Read the model definition and answer for the solid it produces. Units are mm, in the model's axes. A direction names the side the tool comes from. Give positions to 0.01 mm unless a question says otherwise; leave off trailing zeros. Write each loop counter-clockwise with the first axis right and the second up, starting at its lowest first coordinate (ties: lowest second). Pieces come first, ordered by that corner, then holes.
```python
from build123d import *

# Parameters (mm, degrees)
BOSS_EXTRUDE1_DEPTH = 1.5
SKETCH3_W           = 9.15
SKETCH3_H           = 19
CUT_EXTRUDE1_DEPTH  = 1.5
SKETCH2_W           = 33.8
SKETCH2_H           = 1.5
BOSS_EXTRUDE2_DEPTH = 21.85
SKETCH4_R           = 1.5
CUT_EXTRUDE2_DEPTH  = 1.5
BOSS_EXTRUDE3_DEPTH = 1.5
CUT_EXTRUDE4_REACH  = 72.71
SKETCH6_R           = 1.5
SKETCH6_3_R         = 4
CUT_EXTRUDE5_DEPTH  = 1.5
SKETCH8_W           = 24
SKETCH8_H           = 23
BOSS_EXTRUDE5_DEPTH = 1.5
SKETCH9_W           = 8.5
SKETCH9_H           = 8.5
BOSS_EXTRUDE6_DEPTH = 2.7


with BuildPart() as part:
    # Sketch1 → Boss-Extrude1 (new body)
    with BuildSketch(Plane.XY):
        Polygon((-16.9, 0), (16.9, 0), (16.9, 4), (19.2, 4), (19.2, 30), (16.9, 30), (16.9, 34), (13, 34), (13, 36.4), (-13, 36.4), (-13, 34), (-16.9, 34), (-16.9, 30), (-19.2, 30), (-19.2, 4), (-16.9, 4), align=None)
    extrude(amount=BOSS_EXTRUDE1_DEPTH)

    # Sketch3 → Cut-Extrude1 (cut)
    with BuildSketch(Plane.XY.offset(1.5)):
        with Locations((0.125, 21.5)):
            Rectangle(SKETCH3_W, SKETCH3_H)
    extrude(amount=-CUT_EXTRUDE1_DEPTH, mode=Mode.SUBTRACT)

    # Sketch2 → Boss-Extrude2 (add)
    with BuildSketch(Plane(origin=(0, 0, 0), x_dir=(-1, 0, 0), z_dir=(0, 0, -1))):
        with Locations((0, 35.65)):
            Rectangle(SKETCH2_W, SKETCH2_H)
    extrude(amount=BOSS_EXTRUDE2_DEPTH)

    # Sketch4 → Cut-Extrude2 (cut)
    with BuildSketch(Plane(origin=(0, 36.4, 0), x_dir=(1, 0, 0), z_dir=(0, 1, 0))):
        with Locations(Location((-11, 11.7, 0), (0, 0, 270))):
            Circle(SKETCH4_R)
        with Locations(Location((0, 11.7, 0), (0, 0, 270))):
            Circle(SKETCH4_R)
        with Locations(Location((11, 11.7, 0), (0, 0, 270))):
            Circle(SKETCH4_R)
        with BuildLine():
            Line((-11.9, 8.25), (11.9, 8.25))
            ThreePointArc((11.9, 8.25), (13.4, 6.75), (11.9, 5.25))
            Line((11.9, 5.25), (-11.9, 5.25))
            ThreePointArc((-11.9, 5.25), (-13.4, 6.75), (-11.9, 8.25))
        make_face()
        with BuildLine():
            Line((-11.9, 18.15), (11.9, 18.15))
            ThreePointArc((11.9, 18.15), (13.4, 16.65), (11.9, 15.15))
            Line((11.9, 15.15), (-11.9, 15.15))
            ThreePointArc((-11.9, 15.15), (-13.4, 16.65), (-11.9, 18.15))
        make_face()
    extrude(amount=-CUT_EXTRUDE2_DEPTH, mode=Mode.SUBTRACT)

    # Sketch5 → Boss-Extrude3 (add)
    with BuildSketch(Plane(origin=(19.2, 0, 0), x_dir=(0, 0, -1), z_dir=(1, 0, 0))):
        Polygon((0, 30), (0.75, 30), (0.75, 34), (13.17, 46.3), (37.17, 46.3), (37.17, 20.3), (19.75, 0), (0.75, 0), (0.75, 4), (0, 4), (-1.5, 4), (-1.5, 30), align=None)
    boss_extrude3 = extrude(amount=-BOSS_EXTRUDE3_DEPTH)

    # Mirror1: Boss-Extrude3 across plane
    add(boss_extrude3.mirror(Plane(origin=(0, 0, 0), x_dir=(0, 0, 1), z_dir=(1, 0, 0))))

    # Cut-Extrude4: up to this face of the body (flat: up to its plane)
    cut_extrude4_end = Plane(part.part.faces().sort_by_distance((-19.2, 23.875362989, -17.45186466))[0])
    # Sketch6 → Cut-Extrude4 (cut, up to the picked face)
    with BuildSketch(Plane(origin=(19.2, 0, 0), x_dir=(0, 0, -1), z_dir=(1, 0, 0)), mode=Mode.PRIVATE) as cut_extrude4_sk1:
        with Locations((16.67, 42.3)):
            Circle(SKETCH6_R)
    cut_extrude4_tool1 = split(extrude(cut_extrude4_sk1.sketch, amount=-CUT_EXTRUDE4_REACH, mode=Mode.PRIVATE), bisect_by=cut_extrude4_end, keep=Keep.BOTH, mode=Mode.PRIVATE)
    # Sketch6 → Cut-Extrude4 (cut, up to the picked face)
    with BuildSketch(Plane(origin=(19.2, 0, 0), x_dir=(0, 0, -1), z_dir=(1, 0, 0)), mode=Mode.PRIVATE) as cut_extrude4_sk2:
        with Locations((24.67, 42.3)):
            Circle(SKETCH6_R)
    cut_extrude4_tool2 = split(extrude(cut_extrude4_sk2.sketch, amount=-CUT_EXTRUDE4_REACH, mode=Mode.PRIVATE), bisect_by=cut_extrude4_end, keep=Keep.BOTH, mode=Mode.PRIVATE)
    # Sketch6 → Cut-Extrude4 (cut, up to the picked face)
    with BuildSketch(Plane(origin=(19.2, 0, 0), x_dir=(0, 0, -1), z_dir=(1, 0, 0)), mode=Mode.PRIVATE) as cut_extrude4_sk3:
        with Locations((32.67, 42.3)):
            Circle(SKETCH6_R)
    cut_extrude4_tool3 = split(extrude(cut_extrude4_sk3.sketch, amount=-CUT_EXTRUDE4_REACH, mode=Mode.PRIVATE), bisect_by=cut_extrude4_end, keep=Keep.BOTH, mode=Mode.PRIVATE)
    add(cut_extrude4_tool1.solids().sort_by(Axis((19.2, 42.3, -16.67), (-1, 0, 0)))[0], mode=Mode.SUBTRACT)
    add(cut_extrude4_tool2.solids().sort_by(Axis((19.2, 42.3, -24.67), (-1, 0, 0)))[0], mode=Mode.SUBTRACT)
    add(cut_extrude4_tool3.solids().sort_by(Axis((19.2, 42.3, -32.67), (-1, 0, 0)))[0], mode=Mode.SUBTRACT)

    # Sketch6<3> → Cut-Extrude5 (cut)
    with BuildSketch(Plane(origin=(19.2, 0, 0), x_dir=(0, 0, -1), z_dir=(1, 0, 0))):
        with Locations((23.037930183, 16.5)):
            Circle(SKETCH6_3_R)
    extrude(amount=-CUT_EXTRUDE5_DEPTH, mode=Mode.SUBTRACT)

    # Sketch8 → Boss-Extrude5 (add)
    with BuildSketch(Plane(origin=(0, 0, 0), x_dir=(-1, 0, 0), z_dir=(0, 0, -1))):
        with Locations((-0.7, 20)):
            Rectangle(SKETCH8_W, SKETCH8_H)
    extrude(amount=BOSS_EXTRUDE5_DEPTH)

    # Sketch9 → Boss-Extrude6 (add)
    with BuildSketch(Plane.XY):
        with Locations((0.097336639, 16.75)):
            Rectangle(SKETCH9_W, SKETCH9_H)
    extrude(amount=BOSS_EXTRUDE6_DEPTH)


solid = part.part
```
Item 1: Determine the mould class of faces 1 (the flat face through (-16.9, 32, 1)), 2 (the flat face through (0, 36, -21.85)), 3 (the cylindrical face through (-13.4, 35.7, -16.6)) for opening direction Z: pulls with the +Z half, pulls with the -Z half, needs draft (parallel to the pull), parting line crosses it, or undercut.
Result set:
face 1: needs draft
face 2: pulls with the -Z half
face 3: undercut
Item 2: Section B-B (z = -24) is taken. Write down the section's boundary in (x, y).
Result set:
outline: (-19.2, 4.95) - (-17.7, 4.95) - (-17.7, 40.96) - (-19.2, 40.96) - close; (-19.2, 43.64) - (-17.7, 43.64) - (-17.7, 46.3) - (-19.2, 46.3) - close; (17.7, 4.95) - (19.2, 4.95) - (19.2, 12.62) - (17.7, 12.62) - close; (17.7, 20.38) - (19.2, 20.38) - (19.2, 40.96) - (17.7, 40.96) - close; (17.7, 43.64) - (19.2, 43.64) - (19.2, 46.3) - (17.7, 46.3) - close
Item 3: Find the intervals of material crossed by line 1 along X through (y, z) = (35.25, -11.7); line 2 along X through (y, z) = (15, -29); line 3 along Y through (x, z) = (18.35, -16.67), in increasing order.
Result set:
line 1: x = -19.2 to -17.7, -16.9 to -12.5, -9.5 to -1.5, 1.5 to 9.5, 12.5 to 16.9, 17.7 to 19.2
line 2: x = -19.2 to -17.7, 17.7 to 19.2
line 3: y = 0 to 40.8, 43.8 to 46.3
Item 4: Section A-A (x = 7.5) is taken. Write down the section's boundary in (y, z).
Result set:
outline: (0, 0) - (8.5, 0) - (8.5, -1.5) - (31.5, -1.5) - (31.5, 0) - (34.9, 0) - (34.9, -5.25) - (36.4, -5.25) - (36.4, 1.5) - (0, 1.5) - close; (34.9, -21.85) - (36.4, -21.85) - (36.4, -18.15) - (34.9, -18.15) - close; (34.9, -15.15) - (36.4, -15.15) - (36.4, -8.25) - (34.9, -8.25) - close
Item 5: Section C-C (y = 42.3) is taken. Give the number of separate pieces and of enclosed holes in the cut face, and give its area (3 significant figures).
Result set:
separate pieces: 8
enclosed holes: 0
area: 57.1 mm2
Item 6: Section D-D (z = -32.67) is taken. Write down the section's boundary in (x, y).
Result set:
outline: (-19.2, 15.06) - (-17.7, 15.06) - (-17.7, 40.8) - (-19.2, 40.8) - close; (-19.2, 43.8) - (-17.7, 43.8) - (-17.7, 46.3) - (-19.2, 46.3) - close; (17.7, 15.06) - (19.2, 15.06) - (19.2, 40.8) - (17.7, 40.8) - close; (17.7, 43.8) - (19.2, 43.8) - (19.2, 46.3) - (17.7, 46.3) - close
Item 7: Which of the six approach directions +Z, -Z, +X, -X, +Y, -Y give full straight-line access (tool end or side, diameter ignored) to faces 4 (the flat face through (18, 4, 0)), 5 (the cylindrical face through (13.4, 35.7, -16.7)), 6 (the flat face through (0, 21, 1))?
Result set:
face 4: +Z, +X, -Y
face 5: +Y, -Y
face 6: +Z
Item 8: Each of these flat-tipped pins is pushed along its axis until it touches: pin 1 Ø1.6 at (y, z) = (32.5, 1) entering from +X; pin 2 Ø1.2 at (x, z) = (-4, -0.5) entering from +Y; pin 3 Ø5 at (y, z) = (42.3, -24.67) entering from +X; pin 4 Ø1.1 at (x, z) = (17.5, 0) entering from +Y. Where does it stop, or does it pass through?
Result set:
pin 1: stops at x = 16.9
pin 2: stops at y = 36.4
pin 3: stops at x = 19.2
pin 4: stops at y = 30
